```python
from build123d import *

# Parameters (mm, degrees)
F0_W     = 228.6
F0_H     = 558.8
F1_DEPTH = 25.4
F2_W     = 228.6
F2_H     = 25.4
F3_DEPTH = 6.35
F4_W     = 228.6
F4_H     = 25.4
F5_DEPTH = 6.35
F6_R     = 12.7


with BuildPart() as f1:
    # F0 (on Top) → F1 (new body)
    with BuildSketch(Plane.XY):
        Rectangle(F0_W, F0_H)
    extrude(amount=F1_DEPTH)

    # F2 (on face) → F3 (cut)
    with BuildSketch(Plane(origin=(0, 0, 0), x_dir=(1, 0, 0), z_dir=(0, 0, -1))):
        with Locations((0, 241.3)):
            Rectangle(F2_W, F2_H)
    extrude(amount=-F3_DEPTH, mode=Mode.SUBTRACT)

    # F4 (on face) → F5 (cut)
    with BuildSketch(Plane(origin=(0, 0, 0), x_dir=(1, 0, 0), z_dir=(0, 0, -1))):
        with Locations((0, -241.3)):
            Rectangle(F4_W, F4_H)
    extrude(amount=-F5_DEPTH, mode=Mode.SUBTRACT)

    # F6
    f6_edges = [f1.edges().sort_by_distance(p)[0] for p in [
        (0, -279.4, 0),
        (0, 279.4, 0),
    ]]
    fillet(f6_edges, radius=F6_R)


solid = f1.part
```
Verification items for the finished model (mm, model axes). Coordinates: 2 decimals unless noted, no trailing zeros. Loops run counter-clockwise (first coordinate to the right, second up) from the corner with the lowest first, then second, coordinate; pieces in that order, holes last. Notation, with made-up numbers: (-36, 4) - (12, 4) arc R37 cw to (12, 41) - close; hole circle Ø5 at (7, 52). An arc over 180 degrees is marked (long way). Answer as a JSON object with one key per item and string values.
(1) Go/stop test with flat-tipped pins: pin 1 Ø1.9 at (x, z) = (35, 4.5) entering from +Y; pin 2 Ø1.9 at (x, z) = (22, 3.5) entering from +Y; pin 3 Ø5 at (x, z) = (-50.5, 3) entering from -Y. Record where each tip stops, or that it passes through.
Response:
{"pin 1": "stops at y = 277.13", "pin 2": "stops at y = 276.36", "pin 3": "stops at y = -277.16"}
(2) Scan lines: line 1 along Y through (x, z) = (-100, 6); line 2 along Y through (x, z) = (-76, 5); line 3 along Y through (x, z) = (8, 8.5). Record each from-to range of solid material in increasing order.
Response:
{"line 1": "y = -277.49 to -254, -228.6 to 228.6, 254 to 277.49", "line 2": "y = -276.8 to -254, -228.6 to 228.6, 254 to 276.8", "line 3": "y = -278.69 to 278.69"}
(3) Mould release check, pull along Y, two halves, no side actions. Record for faces 1 (the flat face through (-2, -241, 6.35)), 2 (the flat face through (-2, -279.4, 19)), 3 (the flat face through (-2, 241, 6.35)), 4 (the flat face through (-2, 4, 25.4)): pulls with the +Y half, pulls with the -Y half, needs draft (parallel to the pull), parting line crosses it, or undercut.
Response:
{"face 1": "undercut", "face 2": "pulls with the -Y half", "face 3": "undercut", "face 4": "needs draft"}
(4) Cross-section at A-A, the plane x = 82.5. Record the boundary of the cut face in (y, z), then the cut area to 3 significant figures.
Response:
{"outline": "(-279.4, 12.7) arc R12.7 ccw to (-266.7, 0) - (-254, 0) - (-254, 6.35) - (-228.6, 6.35) - (-228.6, 0) - (228.6, 0) - (228.6, 6.35) - (254, 6.35) - (254, 0) - (266.7, 0) arc R12.7 ccw to (279.4, 12.7) - (279.4, 25.4) - (-279.4, 25.4) - close", "area": "13,800 mm²"}
